```python
from build123d import *

# Parameters (mm, degrees)
SKETCH1_W                               = 19
SKETCH1_H                               = 40
SKETCH1_R                               = 4
BOSS_EXTRUDE1_DEPTH                     = 10
CBORE_FOR_M5_HEX_HEAD_BOLT1_D           = 5.5
CBORE_FOR_M5_HEX_HEAD_BOLT1_DEPTH       = 10
CBORE_FOR_M5_HEX_HEAD_BOLT1_CBORE_D     = 12.24
CBORE_FOR_M5_HEX_HEAD_BOLT1_CBORE_DEPTH = 3.58


with BuildPart() as part:
    # Sketch1 → Boss-Extrude1 (new body)
    with BuildSketch(Plane(origin=(0, 0, 0), x_dir=(1, 0, 0), z_dir=(0, 1, 0))):
        Rectangle(SKETCH1_W, SKETCH1_H)
        Circle(SKETCH1_R, mode=Mode.SUBTRACT)
    extrude(amount=BOSS_EXTRUDE1_DEPTH)

    # CBORE for M5 Hex Head Bolt1
    with Locations(Plane(origin=(0, 10, 0), x_dir=(1, 0, 0), z_dir=(0, 1, 0))):
        with Locations((0, 12.5), (0, -12.5)):
            CounterBoreHole(CBORE_FOR_M5_HEX_HEAD_BOLT1_D / 2, CBORE_FOR_M5_HEX_HEAD_BOLT1_CBORE_D / 2, CBORE_FOR_M5_HEX_HEAD_BOLT1_CBORE_DEPTH, depth=CBORE_FOR_M5_HEX_HEAD_BOLT1_DEPTH)


solid = part.part
```
The listing builds one solid part. Answer for the finished solid, in the listing's coordinates (mm). A direction names the side the tool comes from. Coordinates: 2 decimals unless noted, no trailing zeros. Loops run counter-clockwise (first coordinate to the right, second up) from the corner with the lowest first, then second, coordinate; pieces in that order, holes last. Notation, with made-up numbers: M 23.25,56 L 53.25,56 A27 ccw 53.25,81 Z; hole C 88,62.5 d7. An arc over 180 degrees is marked long. Answer as a JSON object with one key per item and string values. Group by question number.
Item 1: Section B-B (y = 8.25) is taken. Write down the section's boundary in (x, z).
Item 2: Section C-C (x = 0) is taken. Write down the section's boundary in (y, z), and give its area (3 significant figures).
Item 3: Section D-D (y = 5.75) is taken. Write down the section's boundary in (x, z), and give its area (3 significant figures).
Item 4: Section A-A (z = 12.5) is taken. Write down the section's boundary in (x, y).
Item 5: Consider L1, parallel to Z at x = 0, y = 3; L2, parallel to X at y = 6.25, z = 0; L3, parallel to Z at x = 0, y = 9.05. Determine where each line is inside the solid, lowest interval first.
Item 6: Which of the six approach directions +Z, -Z, +X, -X, +Y, -Y give full straight-line access (tool end or side, diameter ignored) to faces 1 (the face through (0, 5, -20)), 2 (the face through (3, 6.42, -11))?
Item 7: Determine the mould class of faces 3 (the face through (-4.511, 8.235, -16.636)), 4 (the face through (3, 6.42, 14)), 5 (the face through (-4.4, 0, -0.3)), 6 (the face through (9.5, 5, 0)) for opening direction X: +X half, -X half, draft (parallel to the pull), parting line (faces both ways), or undercut.
Item 8: This flat-tipped pin is pushed along its axis until it touches: P1, Ø6, axis at x = -1.5, z = -12, coming from the +Y side. Where does it stop, or does it pass through?
Solved:
{
 "1": {"outline": "M -9.5,-20 L 9.5,-20 L 9.5,20 L -9.5,20 Z; hole C 0,-12.5 d12.24; hole C 0,12.5 d12.24; hole C 0,0 d8"},
 "2": {"outline": "M 0,-20 L 10,-20 L 10,-18.62 L 6.42,-18.62 L 6.42,-15.25 L 0,-15.25 Z; M 0,-9.75 L 6.42,-9.75 L 6.42,-6.38 L 10,-6.38 L 10,-4 L 0,-4 Z; M 0,4 L 10,4 L 10,6.38 L 6.42,6.38 L 6.42,9.75 L 0,9.75 Z; M 0,15.25 L 6.42,15.25 L 6.42,18.62 L 10,18.62 L 10,20 L 0,20 Z", "area": "162 mm2"},
 "3": {"outline": "M -9.5,-20 L 9.5,-20 L 9.5,20 L -9.5,20 Z; hole C 0,0 d8; hole C 0,-12.5 d5.5; hole C 0,12.5 d5.5", "area": "662 mm2"},
 "4": {"outline": "M -9.5,0 L -2.75,0 L -2.75,6.42 L -6.12,6.42 L -6.12,10 L -9.5,10 Z; M 2.75,0 L 9.5,0 L 9.5,10 L 6.12,10 L 6.12,6.42 L 2.75,6.42 Z"},
 "5": {"L1": "z = -20 to -15.25, -9.75 to -4, 4 to 9.75, 15.25 to 20", "L2": "x = -9.5 to -4, 4 to 9.5", "L3": "z = -20 to -18.62, -6.38 to -4, 4 to 6.38, 18.62 to 20"},
 "6": {"face 1": "-Z, +X, -X, +Y, -Y", "face 2": "+Y"},
 "7": {"face 3": "undercut", "face 4": "undercut", "face 5": "draft", "face 6": "+X half"},
 "8": {"P1": "stops at y = 6.42"}
}
